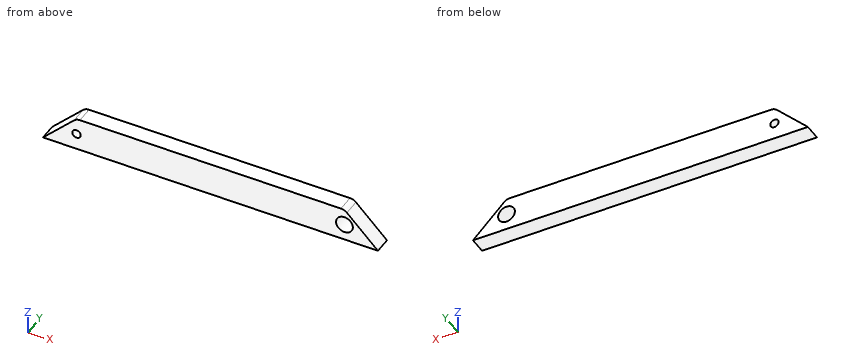
```python
from build123d import *

# Parameters (mm, degrees)
F0_W     = 200
F0_H     = 20
F0_R     = 2.5
F0_R_2   = 5
F1_DEPTH = 5
F2_SIZE  = 19.99999
F3_R     = 5


# Not quite as in the source:
# - a fillet or chamfer is up to 0.001 mm smaller than in the source, because OpenCascade refuses the exact size


with BuildPart() as f1:
    # F0 (on Front) → F1 (new body, symmetric)
    with BuildSketch(Plane.XZ):
        with Locations((25, -13.3771840364)):
            Rectangle(F0_W, F0_H)
        with Locations((-55, -13.3771840364)):
            Circle(F0_R, mode=Mode.SUBTRACT)
        with Locations((105, -13.3771840364)):
            Circle(F0_R_2, mode=Mode.SUBTRACT)
    extrude(amount=F1_DEPTH, both=True)

    # F2 (size 20 in the source; OpenCascade refuses exactly that, so slightly less here)
    f2_edges = [f1.edges().sort_by_distance(p)[0] for p in [
        (-75, 0, -3.377184),
        (125, 0, -3.377184),
    ]]
    chamfer(f2_edges, length=F2_SIZE)

    # F3
    f3_edges = [f1.edges().sort_by_distance(p)[0] for p in [
        (-55.00001, 0, -3.377184),
        (105.00001, 0, -3.377184),
    ]]
    fillet(f3_edges, radius=F3_R)


solid = f1.part
```
Input: part model. Units: mm. Frame: model coordinates. Give positions to 0.01 mm unless a question says otherwise; leave off trailing zeros. Order: outer loops, then holes, each group sorted by start corner. A loop starts at its lowest first (then second) coordinate and runs counter-clockwise, first axis right, second up. Notation, with made-up numbers: M 78,83.5 L 122,83.5 A20 cw 122,118.5 Z; hole C 14.25,81.25 d11. An arc over 180 degrees is marked long. One line per question, with ' | ' between items.
1) Section A-A on y = -3.25. State how many separate pieces and enclosed holes the cut face has, and give its area (3 significant figures).
Filled in:
separate pieces: 1 | enclosed holes: 2 | area: 3,500 mm2
2) Ray query, L1, parallel to X at y = -0.5, z = -14; L2, parallel to X at y = 1.5, z = -11.5; L3, parallel to X at y = -3.5, z = -10.25. Return the intervals inside material, ascending.
Filled in:
L1: x = -65.62 to -57.42, -52.58 to 100.04, 109.96 to 115.62 | L2: x = -63.12 to -56.65, -53.35 to 100.37, 109.63 to 113.12 | L3: x = -61.87 to 101.1, 108.9 to 111.87
3) Section B-B on z = -21.25. Output: boundary loops of the cut face in (x, y), and give its area (3 significant figures).
Filled in:
outline: M -72.87,-5 L 122.87,-5 L 122.87,5 L -72.87,5 Z | area: 1,960 mm2
4) Contact query for flat-ended pins moving along their axis: P1, Ø8, axis at x = -55, z = -13.38, coming from the -Y side; P2, Ø1, axis at y = 2.5, z = -17.5, coming from the -X side; P3, Ø6, axis at y = 0, z = -11, coming from the -X side; P4, Ø6, axis at y = 0, z = -6.5, coming from the -X side. Output: stop coordinate, or through.
Filled in:
P1: stops at y = -5 | P2: stops at x = -69.62 | P3: stops at x = -65.62 | P4: stops at x = -61.12
